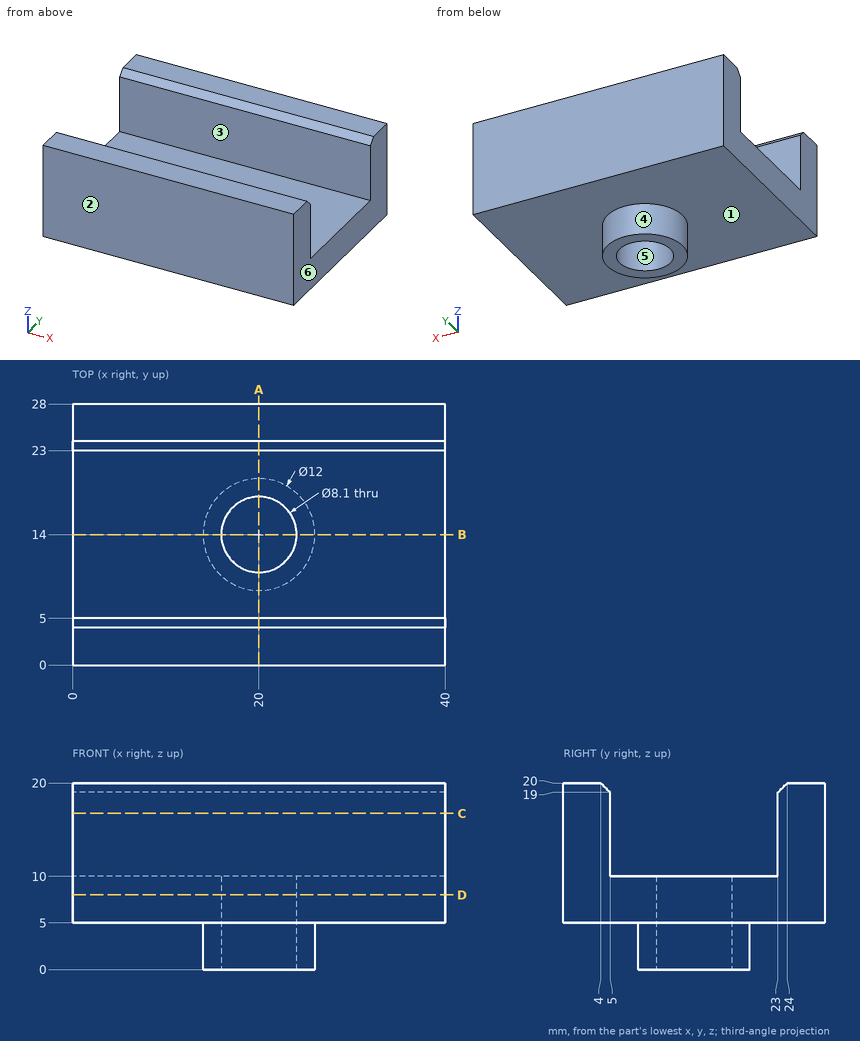
Print and shaded views of the part. All mm, measured from the part's lowest x, y and z. A direction names the side the tool comes from. Give positions to 0.01 mm unless a question says otherwise; leave off trailing zeros. Write each loop counter-clockwise with the first axis right and the second up, starting at its lowest first coordinate (ties: lowest second). Pieces come first, ordered by that corner, then holes. Notation, with made-up numbers: (45.5, 88) - (97.5, 88) arc R12 cw to (97.5, 92) - close; hole circle Ø8 at (21.25, 59). An arc over 180 degrees is marked (long way). One line per question, with ' | ' between items. Start each with the question number.
(1) Two-plate mould, pull along Y, no slides. Class the marked faces 4, 5 and 6: +Y half, -Y half, draft (parallel to the pull), parting line (faces both ways), or undercut.
(2) Slice it at B-B on y = 14. Write the cut outline in (x, z).
(3) Slice it at D-D on z = 8. Write the cut outline in (x, y), plus the area to 3 significant figures.
(4) Pin check, flat tips, straight feed: P1, Ø10, axis at y = 9.5, z = 9.5, coming from the -X side; P2, Ø4, axis at x = 7, y = 3, coming from the -Z side. Stop position of each tip, or through.
(5) Wall check: line 1 along Y through (x, z) = (18, 12); line 2 along Y through (x, z) = (20, 7.25); line 3 along Z through (x, y) = (21, 24.25). Give the ranges that are in metal, low to high. Write a range as from..to.
(6) Slice it at C-C on z = 16.75. Write the cut outline in (x, y), plus the area to 3 significant figures.
(7) Slice it at A-A on x = 20. Write the cut outline in (y, z), plus the area to 3 significant figures.
(8) 3-axis set-ups, long thin cutter, end or side, ignore diameter. For the marked faces 1, 2 and 3: which of +Z, -Z, +X, -X, +Y, -Y reach the whole face in a straight line?
Results below:
1) face 4: parting line | face 5: undercut | face 6: draft
2) outline: (0, 5) - (14, 5) - (14, 0) - (15.95, 0) - (15.95, 10) - (0, 10) - close; (24.05, 0) - (26, 0) - (26, 5) - (40, 5) - (40, 10) - (24.05, 10) - close
3) outline: (0, 0) - (40, 0) - (40, 28) - (0, 28) - close; hole circle Ø8.1 at (20, 14) | area: 1,070 mm^2
4) P1: x = 0 | P2: z = 5
5) line 1: 0..5, 23..28 | line 2: 0..9.95, 18.05..28 | line 3: 5..20
6) outline: (0, 0) - (40, 0) - (40, 5) - (0, 5) - close; (0, 23) - (40, 23) - (40, 28) - (0, 28) - close | area: 400 mm^2
7) outline: (0, 5) - (8, 5) - (8, 0) - (9.95, 0) - (9.95, 10) - (5, 10) - (5, 19) - (4, 20) - (0, 20) - close; (18.05, 0) - (20, 0) - (20, 5) - (28, 5) - (28, 20) - (24, 20) - (23, 19) - (23, 10) - (18.05, 10) - close | area: 218 mm^2
8) face 1: -Z | face 2: +Z, -Z, +X, -X, -Y | face 3: +Z, +X, -X
